Can you work these out from the model? Positions are in its coordinate system, mm. Face numbers are marked on the shaded views. A direction names the side the tool comes from. Give positions to 0.01 mm unless a question says otherwise; leave off trailing zeros. Order: outer loops, then holes, each group sorted by start corner. A loop starts at its lowest first (then second) coordinate and runs counter-clockwise, first axis right, second up. Notation, with made-up numbers: (82.25, 18) -> (131.25, 18) arc R14 cw to (131.25, 40) -> close; hole circle Ø2 at (87.5, 83). An arc over 180 degrees is marked (long way). Answer as CSV lines item,"result".
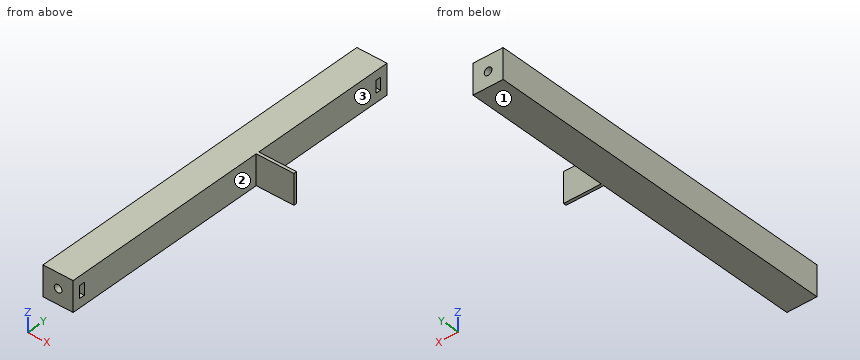
```python
from build123d import *

# Parameters (mm, degrees)
ESQUISSE1_W             = 20
ESQUISSE1_H             = 20
BOSS_EXTRU_2_DEPTH      = 240
ESQUISSE5_W             = 8.1
ESQUISSE5_H             = 3.5
ENL_V_MAT_EXTRU_2_DEPTH = 10
ESQUISSE6_R             = 2.55
ENL_V_MAT_EXTRU_3_DEPTH = 25
ENL_V_START             = 3.5
ENL_V_MAT_EXTRU_5_DEPTH = 3.5
ENL_V_START_2           = -25
ESQUISSE9_R             = 2.55
ENL_V_MAT_EXTRU_6_DEPTH = 25
ESQUISSE10_W            = 20
ESQUISSE10_H            = 2
BOSS_EXTRU_5_DEPTH      = 25


with BuildPart() as part:
    # Esquisse1 → Boss.-Extru.2 (new body)
    with BuildSketch(Plane(origin=(0, 0, 0), x_dir=(1, 0, 0), z_dir=(0, 1, 0))):
        Rectangle(ESQUISSE1_W, ESQUISSE1_H)
    extrude(amount=BOSS_EXTRU_2_DEPTH)

    # Esquisse5 → Enlèv. mat.-Extru.2 (cut)
    with BuildSketch(Plane(origin=(10, 0, 0), x_dir=(0, 0, -1), z_dir=(1, 0, 0))):
        with Locations((0, 233.25)):
            Rectangle(ESQUISSE5_W, ESQUISSE5_H)
        with Locations((0, 6.75)):
            Rectangle(ESQUISSE5_W, ESQUISSE5_H)
    extrude(amount=-ENL_V_MAT_EXTRU_2_DEPTH, mode=Mode.SUBTRACT)

    # Esquisse6 → Enlèv. mat.-Extru.3 (cut)
    with BuildSketch(Plane(origin=(0, 240, 0), x_dir=(1, 0, 0), z_dir=(0, 1, 0))):
        with Locations(Location((0, 0, 0), (0, 0, 270))):
            Circle(ESQUISSE6_R)
    extrude(amount=-ENL_V_MAT_EXTRU_3_DEPTH, mode=Mode.SUBTRACT)

    # Esquisse7 → Enlèv. mat.-Extru.5 (cut)
    with BuildSketch(Plane(origin=(0, 231.5, 0), x_dir=(1, 0, 0), z_dir=(0, 1, 0)).offset(ENL_V_START)):
        with BuildLine():
            Line((-2.33826859, -4.05), (0, -4.05))
            Line((0, -4.05), (0, -2.55))
            ThreePointArc((0, -2.55), (-2.55, 0), (0, 2.55))
            Line((0, 2.55), (0, 4.05))
            Line((0, 4.05), (-2.33826859, 4.05))
            Line((-2.33826859, 4.05), (-4.67653718, 0))
            Line((-4.67653718, 0), (-2.33826859, -4.05))
        make_face()
    extrude(amount=-ENL_V_MAT_EXTRU_5_DEPTH, mode=Mode.SUBTRACT)

    # Esquisse9 → Enlèv. mat.-Extru.6 (cut)
    with BuildSketch(Plane.XZ.offset(ENL_V_START_2)):
        with Locations(Location((0, 0, 0), (0, 0, 90))):
            Circle(ESQUISSE9_R)
    extrude(amount=ENL_V_MAT_EXTRU_6_DEPTH, mode=Mode.SUBTRACT)

    # Esquisse10 → Boss.-Extru.5 (add)
    with BuildSketch(Plane(origin=(10, 0, 0), x_dir=(0, 0, -1), z_dir=(1, 0, 0))):
        with Locations((0, 141)):
            Rectangle(ESQUISSE10_W, ESQUISSE10_H)
    extrude(amount=BOSS_EXTRU_5_DEPTH)


solid = part.part
```
Item 1: For the marked faces 1, 2 and 3, which set-ups out of +Z, -Z, +X, -X, +Y, -Y let a thin tool reach every point of the face, with its end or its side?
Numbers:
face 1,"-Z, +X, -X, +Y, -Y"
face 2,"+Z, -Z, +X, -Y"
face 3,"+Z, -Z, +X, +Y"
Item 2: Please list where these lines run through material, in increasing order: line 1 along X through (y, z) = (14.75, 0); line 2 along Y through (x, z) = (2.5, 2.5).
Numbers:
line 1,"x = -10 to -2.55, 2.55 to 10"
line 2,"y = 0 to 5, 8.5 to 231.5, 235 to 240"
Item 3: Imagine slicing it at A-A, the plane z = 7. Please give me the cut outline in (x, y), then the cut area to 3 significant figures.
Numbers:
outline,"(-10, 0) -> (10, 0) -> (10, 140) -> (35, 140) -> (35, 142) -> (10, 142) -> (10, 240) -> (-10, 240) -> close"
area,"4,850 mm²"
Item 4: Imagine slicing it at B-B, the plane y = 136.5. Please give me the cut outline in (x, z), then the cut area to 3 significant figures.
Numbers:
outline,"(-10, -10) -> (10, -10) -> (10, 10) -> (-10, 10) -> close"
area,"400 mm²"
Item 5: Imagine slicing it at C-C, the plane x = 26. Please give me the cut outline in (y, z), then the cut area to 3 significant figures.
Numbers:
outline,"(140, -10) -> (142, -10) -> (142, 10) -> (140, 10) -> close"
area,"40.0 mm²"
Item 6: For pin 1 (5 mm diameter, centred on x = 14.5, y = 200, fed in from +Z); pin 2 (6 mm diameter, centred on y = 95.5, z = -3.5, fed in from +X); pin 3 (1.5 mm diameter, centred on x = 20.5, z = 7, fed in from +Y); pin 4 (1.5 mm diameter, centred on x = -0.5, z = 0, fed in from +Y), each with a flat end and sliding along its axis, tell me the tip position at first contact or that it passes through.
Numbers:
pin 1,"passes through"
pin 2,"stops at x = 10"
pin 3,"stops at y = 142"
pin 4,"stops at y = 215"
